Part model, mm, in its own coordinate system. Round coordinates to 2 decimals unless told otherwise and drop trailing zeros. Loops run counter-clockwise (first coordinate to the right, second up) from the corner with the lowest first, then second, coordinate; pieces in that order, holes last.
(1) Cut at D-D on x = -295. List the corners of the cut face in (y, z), then the cut area to 3 significant figures.
(2) Cut at B-B on x = -68.5. List the corners of the cut face in (y, z).
(3) Cut at C-C on y = 235. List the corners of the cut face in (x, z).
(4) Cut at A-A on y = -181. List the corners of the cut face in (x, z), then the cut area to 3 significant figures.
(5) Flat gauge pins, fed straight in: pin 1 (3 mm diameter, centred on y = 116, z = 5, fed in from +X); pin 2 (2 mm diameter, centred on y = 266, z = 4.5, fed in from +X); pin 3 (4 mm diameter, centred on y = -149.5, z = 6, fed in from -X). Where does each tip first touch, or does it go through?
(6) Probe probe 1 along Y at (x, z) = (0, 2.75); probe 2 along X at (y, z) = (120.5, 12); probe 3 along X at (y, z) = (249.5, 9). List the from-to ranges inside material, lowest first.
from build123d import *

# Parameters (mm, degrees)
SKETCH_R           = 375
SKETCH_R_2         = 12.5
PAD_DEPTH          = 12.7
POCKET_DEPTH       = 12.7
POLARPATTERN_COUNT = 11


with BuildPart() as part:
    # Sketch → Pad (new body)
    with BuildSketch(Plane.XY):
        Circle(SKETCH_R)
        Circle(SKETCH_R_2, mode=Mode.SUBTRACT)
    extrude(amount=PAD_DEPTH)

    # Sketch001 (on Face4 of Pad) → Pocket (cut)
    with BuildSketch(Plane.XY.offset(12.7)):
        with BuildLine():
            ThreePointArc((52.416839, 272.99275), (0, 337.5), (-52.416839, 272.99275))
            Line((-52.416839, 272.99275), (-6.988912, 55.679))
            ThreePointArc((-6.988912, 55.679), (0, 50), (6.988912, 55.679))
            Line((52.416839, 272.99275), (6.988912, 55.679))
        make_face()
    pocket = extrude(amount=-POCKET_DEPTH, mode=Mode.SUBTRACT)

    # PolarPattern: Pocket ×11 about axis
    polarpattern_axis = Axis((0, 0, 12.7), (0, 0, 1))
    for i in range(1, POLARPATTERN_COUNT):
        add(pocket.rotate(polarpattern_axis, i * 360 / POLARPATTERN_COUNT), mode=Mode.SUBTRACT)


solid = part.part
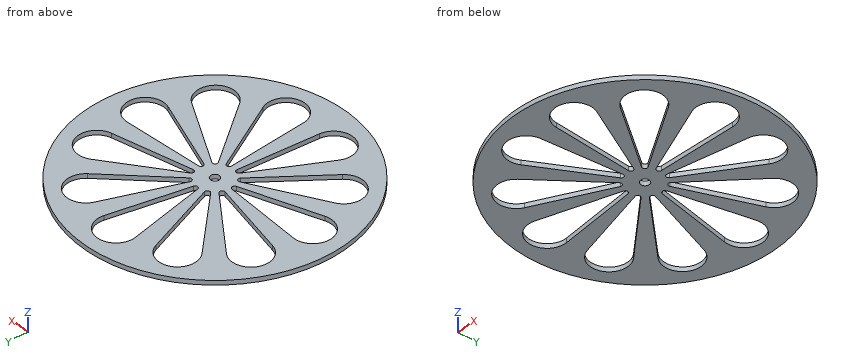
Final values:
1. outline: (-231.52, 0) - (-92.11, 0) - (-92.11, 12.7) - (-231.52, 12.7) - close; (11.29, 0) - (78.97, 0) - (78.97, 12.7) - (11.29, 12.7) - close; (156.94, 0) - (231.52, 0) - (231.52, 12.7) - (156.94, 12.7) - close
1. area: 3,580 mm2
2. outline: (-368.69, 0) - (-324.75, 0) - (-324.75, 12.7) - (-368.69, 12.7) - close; (-137.55, 0) - (-82.46, 0) - (-82.46, 12.7) - (-137.55, 12.7) - close; (-43.34, 0) - (-20.07, 0) - (-20.07, 12.7) - (-43.34, 12.7) - close; (-0.22, 0) - (20.15, 0) - (20.15, 12.7) - (-0.22, 12.7) - close; (44.76, 0) - (76.11, 0) - (76.11, 12.7) - (44.76, 12.7) - close; (166.45, 0) - (368.69, 0) - (368.69, 12.7) - (166.45, 12.7) - close
3. outline: (-292.23, 0) - (-206.92, 0) - (-206.92, 12.7) - (-292.23, 12.7) - close; (-94.71, 0) - (-44.47, 0) - (-44.47, 12.7) - (-94.71, 12.7) - close; (44.47, 0) - (94.71, 0) - (94.71, 12.7) - (44.47, 12.7) - close; (206.92, 0) - (292.23, 0) - (292.23, 12.7) - (206.92, 12.7) - close
4. outline: (-328.43, 0) - (-267.92, 0) - (-267.92, 12.7) - (-328.43, 12.7) - close; (-143.52, 0) - (-91.77, 0) - (-91.77, 12.7) - (-143.52, 12.7) - close; (-18.99, 0) - (18.99, 0) - (18.99, 12.7) - (-18.99, 12.7) - close; (91.77, 0) - (143.52, 0) - (143.52, 12.7) - (91.77, 12.7) - close; (267.92, 0) - (328.43, 0) - (328.43, 12.7) - (267.92, 12.7) - close
4. area: 3,330 mm2
5. pin 1: stops at x = 357.09
5. pin 2: stops at x = 265.33
5. pin 3: stops at x = -344.77
6. probe 1: y = -375 to -12.5, 12.5 to 50, 337.5 to 375
6. probe 2: x = -355.11 to -311.78, -171.4 to -112.17, -50.94 to -20.54, 20.54 to 50.94, 112.17 to 171.4, 311.78 to 355.11
6. probe 3: x = -279.95 to -206, -100.25 to -47.51, 47.51 to 100.25, 206 to 279.95
